Verification items for the finished model (mm, model axes). A direction names the side the tool comes from. Coordinates: 2 decimals unless noted, no trailing zeros. Order: outer loops, then holes, each group sorted by start corner. A loop starts at its lowest first (then second) coordinate and runs counter-clockwise, first axis right, second up. Notation, with made-up numbers: M -19.75,53.5 L -3.75,53.5 A27 cw -3.75,92.5 Z; hole C 38.5,86 d8. An arc over 180 degrees is marked long. Return JSON: item names as keys, results as strings. Group by question number.
1. Set-up check for faces 1 (the flat face through (-53.315, -16, 31)), 2 (the flat face through (4, 2, 13.081)), 3 (the flat face through (-1, 3, 0)): record each of +Z, -Z, +X, -X, +Y, -Y from which the full face is reachable in a straight line by a thin tool's end or side.
2. Section check D-D, the plane y = -27.5. Record the cut outline in (x, z) (3 decimals).
3. Section check B-B, the plane x = 34. Record the cut outline in (y, z) (3 decimals), plus the area to 3 significant figures.
4. Gauge pin test, flat ends, axial feed: pin 1 (4 mm diameter, centred on x = 50.038, z = -20.447, fed in from +Y); pin 2 (1 mm diameter, centred on y = -13, z = 31.5, fed in from +X); pin 3 (6 mm diameter, centred on x = 40.5, y = -28, fed in from -Z) (3 decimals); pin 4 (2 mm diameter, centred on x = 50.038, z = 20.447, fed in from +Y). Record the tip position at first contact, or that the pin passes through.
5. Mould release check, pull along X, two halves, no side actions. Record for faces 4 (the flat face through (53.315, -16, 31)), 5 (the cylindrical face through (-50.113, 0.786, -22.145)), 6 (the flat face through (-1, -15, 33.147)): +X half, -X half, draft (parallel to the pull), parting line (faces both ways), or undercut.
6. Section check A-A, the plane z = -11. Record the cut outline in (x, y).
7. Section check C-C, the plane z = 15.5. Record the cut outline in (x, y), plus the area to 3 significant figures.
8. Material ranges on line 1 along Z through (x, y) = (43.5, -15.5) (3 decimals); line 2 along Y through (x, z) = (32.5, -23), recorded low to high.
```python
from build123d import *

# Parameters (mm, degrees)
SKETCH1_W                                    = 112.776
SKETCH1_H                                    = 66.294
BOSS_EXTRUDE1_DEPTH                          = 3
CSK_FOR_M3_COUNTERSUNK_FLAT_HEAD_SCR_2_COUNT = 2
CSK_FOR_M3_COUNTERSUNK_FLAT_HEAD_SCR_2_PITCH = 40.894
CSK_FOR_M3_COUNTERSUNK_FLAT_HEAD_SCR_3_COUNT = 2
CSK_FOR_M3_COUNTERSUNK_FLAT_HEAD_SCR_3_PITCH = 108.108857232
CSK_FOR_M3_COUNTERSUNK_FLAT_HEAD_SCR_4_COUNT = 2
CSK_FOR_M3_COUNTERSUNK_FLAT_HEAD_SCR_4_PITCH = 100.076
SKETCH4_W                                    = 106.6292
SKETCH4_H                                    = 3.302
BOSS_EXTRUDE2_DEPTH                          = 31.75
CUT_EXTRUDE1_REACH                           = 76.067
SKETCH6_W                                    = 6.35
SKETCH6_H                                    = 6.35
SKETCH6_W_2                                  = 7.874
SKETCH6_H_2                                  = 8.89


with BuildPart() as part:
    # Sketch1 → Boss-Extrude1 (new body)
    with BuildSketch(Plane(origin=(0, 0, 0), x_dir=(1, 0, 0), z_dir=(0, 1, 0))):
        Rectangle(SKETCH1_W, SKETCH1_H)
    extrude(amount=BOSS_EXTRUDE1_DEPTH)

    # Sketch3 → CSK for M3 Countersunk Flat Head Screw1 (revolve, cut)
    with BuildSketch(Plane(origin=(-50.038, 3, -20.447), x_dir=(0, 0, 1), z_dir=(1, 0, 0))):
        Polygon((0, 0), (0, 3), (1.7, 3), (1.7, 1.45), (3.15, 0), align=None)
    csk_for_m3_countersunk_flat_head_screw1 = revolve(axis=Axis((-50.038, 9.35, -20.447), (0, -1, 0)), mode=Mode.SUBTRACT)

    # CSK for M3 Countersunk Flat Head Scr 2: CSK for M3 Countersunk Flat Head Screw1 ×2
    with Locations(*[(0, 0, i * CSK_FOR_M3_COUNTERSUNK_FLAT_HEAD_SCR_2_PITCH) for i in range(1, CSK_FOR_M3_COUNTERSUNK_FLAT_HEAD_SCR_2_COUNT)]):
        add(csk_for_m3_countersunk_flat_head_screw1, mode=Mode.SUBTRACT)

    # CSK for M3 Countersunk Flat Head Scr 3: CSK for M3 Countersunk Flat Head Screw1 ×2
    with Locations(*[Vector(0.9256965854821381, 0, 0.3782668788391479) * (i * CSK_FOR_M3_COUNTERSUNK_FLAT_HEAD_SCR_3_PITCH) for i in range(1, CSK_FOR_M3_COUNTERSUNK_FLAT_HEAD_SCR_3_COUNT)]):
        add(csk_for_m3_countersunk_flat_head_screw1, mode=Mode.SUBTRACT)

    # CSK for M3 Countersunk Flat Head Scr 4: CSK for M3 Countersunk Flat Head Screw1 ×2
    with Locations(*[(i * CSK_FOR_M3_COUNTERSUNK_FLAT_HEAD_SCR_4_PITCH, 0, 0) for i in range(1, CSK_FOR_M3_COUNTERSUNK_FLAT_HEAD_SCR_4_COUNT)]):
        add(csk_for_m3_countersunk_flat_head_screw1, mode=Mode.SUBTRACT)

    # Sketch4 → Boss-Extrude2 (add)
    with BuildSketch(Plane.XZ):
        with Locations((0, 31.496)):
            Rectangle(SKETCH4_W, SKETCH4_H)
    extrude(amount=BOSS_EXTRUDE2_DEPTH)

    # Sketch6 → Cut-Extrude1 (cut, up to next)
    with BuildSketch(Plane(origin=(0, 3, 0), x_dir=(1, 0, 0), z_dir=(0, 1, 0)), mode=Mode.PRIVATE) as cut_extrude1_sk1:
        with Locations((4.445, -16.256)):
            Rectangle(SKETCH6_W, SKETCH6_H)
    cut_extrude1_tool1 = extrude(cut_extrude1_sk1.sketch, amount=-CUT_EXTRUDE1_REACH, mode=Mode.PRIVATE) & part.part
    # Sketch6 → Cut-Extrude1 (cut, up to next)
    with BuildSketch(Plane(origin=(0, 3, 0), x_dir=(1, 0, 0), z_dir=(0, 1, 0)), mode=Mode.PRIVATE) as cut_extrude1_sk2:
        with Locations((5.207, 9.398)):
            Rectangle(SKETCH6_W_2, SKETCH6_H_2)
    cut_extrude1_tool2 = extrude(cut_extrude1_sk2.sketch, amount=-CUT_EXTRUDE1_REACH, mode=Mode.PRIVATE) & part.part
    add(cut_extrude1_tool1.solids().sort_by_distance((4.445, 3, 16.256))[0], mode=Mode.SUBTRACT)
    add(cut_extrude1_tool2.solids().sort_by_distance((5.207, 3, -9.398))[0], mode=Mode.SUBTRACT)


solid = part.part
```
Answers follow:
{
 "1": {"face 1": "+Z, -Z, -X, -Y", "face 2": "+Y, -Y", "face 3": "+Z, -Z, +X, -X, +Y"},
 "2": {"outline": "M -53.315,29.845 L 53.315,29.845 L 53.315,33.147 L -53.315,33.147 Z"},
 "3": {"outline": "M -31.75,29.845 L 0,29.845 L 0,-33.147 L 3,-33.147 L 3,33.147 L -31.75,33.147 Z", "area": "304 mm^2"},
 "4": {"pin 1": "y = 1.85", "pin 2": "x = 53.31", "pin 3": "z = 29.845", "pin 4": "through"},
 "5": {"face 4": "+X half", "face 5": "undercut", "face 6": "draft"},
 "6": {"outline": "M -56.39,0 L 1.27,0 L 1.27,3 L -56.39,3 Z; M 9.14,0 L 56.39,0 L 56.39,3 L 9.14,3 Z"},
 "7": {"outline": "M -56.39,0 L 1.27,0 L 1.27,3 L -56.39,3 Z; M 7.62,0 L 56.39,0 L 56.39,3 L 7.62,3 Z", "area": "319 mm^2"},
 "8": {"line 1": "29.845 to 33.147", "line 2": "0 to 3"}
}
